Can you work these out from the model? Positions are in its coordinate system, mm. Face numbers are marked on the shaded views. Give positions to 0.01 mm unless a question says otherwise; leave off trailing zeros. Loops run counter-clockwise (first coordinate to the right, second up) from the corner with the lowest first, then second, coordinate; pieces in that order, holes last. Notation, with made-up numbers: M 25,21.5 L 69,21.5 A15 cw 69,34.5 Z; hole C 50.25,58 d3. An arc over 180 degrees is marked long. Use CSV: the item, a comma, the result in double quotes.
from build123d import *

# Parameters (mm, degrees)
F0_W     = 503
F0_H     = 316
F1_DEPTH = 50
F2_R     = 2
F3_DEPTH = 10
F4_W     = 476.64
F4_H     = 268.11
F5_DEPTH = 3


with BuildPart() as f1:
    # F0 (on Top) → F1 (new body)
    with BuildSketch(Plane.XY):
        with Locations((251.5, 158)):
            Rectangle(F0_W, F0_H)
    extrude(amount=F1_DEPTH)

    # F2 (on face) → F3 (cut)
    with BuildSketch(Plane(origin=(0, 0, 0), x_dir=(1, 0, 0), z_dir=(0, 0, -1))):
        with Locations((301.5, -208)):
            Circle(F2_R)
        with Locations((201.5, -208)):
            Circle(F2_R)
        with Locations((201.5, -108)):
            Circle(F2_R)
        with Locations((301.5, -108)):
            Circle(F2_R)
    extrude(amount=-F3_DEPTH, mode=Mode.SUBTRACT)

    # F4 (on face) → F5 (cut)
    with BuildSketch(Plane.XY.offset(50)):
        with Locations((251.5, 158)):
            Rectangle(F4_W, F4_H)
    extrude(amount=-F5_DEPTH, mode=Mode.SUBTRACT)


solid = f1.part
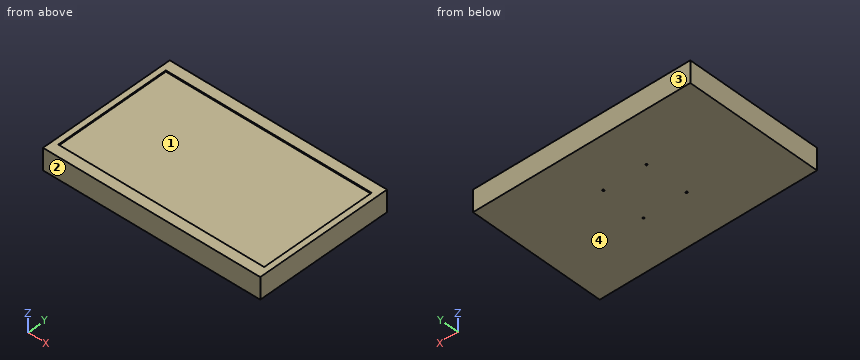
Q1. I'm going to push flat-ended pins straight in: P1, Ø3, axis at x = 201.5, y = 108, coming from the -Z side; P2, Ø1.5, axis at x = 166.5, z = 48, coming from the -Y side; P3, Ø4, axis at x = 146.5, y = 208.5, coming from the +Z side. Where does each tip first touch, or does it pass through?
Model answer:
P1,"z = 10"
P2,"y = 0"
P3,"z = 47"
Q2. If we mould it in two halves opening along Y, with no side actions, what happens to the marked faces 1, 2, 3 and 4? For each: released by +Y, released by -Y, zero draft, split by the parting line, or undercut.
Model answer:
face 1,"undercut"
face 2,"released by -Y"
face 3,"released by +Y"
face 4,"zero draft"
Q3. I want a section at B-B, the plane x = 378. Please give me the cut outline in (y, z) (3 decimals), then the cut area to 3 significant figures.
Model answer:
outline,"M 0,0 L 316,0 L 316,50 L 292.055,50 L 292.055,47 L 23.945,47 L 23.945,50 L 0,50 Z"
area,"15,000 mm2"
Q4. I want a section at A-A, the plane y = 133. Please give me the cut outline in (x, z), then the cut area to 3 significant figures.
Model answer:
outline,"M 0,0 L 503,0 L 503,50 L 489.82,50 L 489.82,47 L 13.18,47 L 13.18,50 L 0,50 Z"
area,"23,700 mm2"
Q5. Please list where these lines run through material, in increasing order: L1, parallel to X at y = 108, z = 5.5; L2, parallel to Y at x = 201.5, z = 2.25; L3, parallel to Y at x = 301, z = 5. Write a range as from..to.
Model answer:
L1,"0..199.5, 203.5..299.5, 303.5..503"
L2,"0..106, 110..206, 210..316"
L3,"0..106.06, 109.94..206.06, 209.94..316"
